Input: part model. Units: mm. Frame: model coordinates. Face numbers are marked on the shaded views. A direction names the side the tool comes from. Round coordinates to 2 decimals unless told otherwise and drop trailing zeros. Order: outer loops, then holes, each group sorted by start corner. A loop starts at its lowest first (then second) coordinate and runs counter-clockwise, first axis right, second up. Notation, with made-up numbers: (38, 22) -> (84, 22) arc R32 ccw to (84, 60) -> close; hole circle Ø1 at (86.5, 6.5). An arc over 180 degrees is marked (long way). Use a Markdown table: item, result.
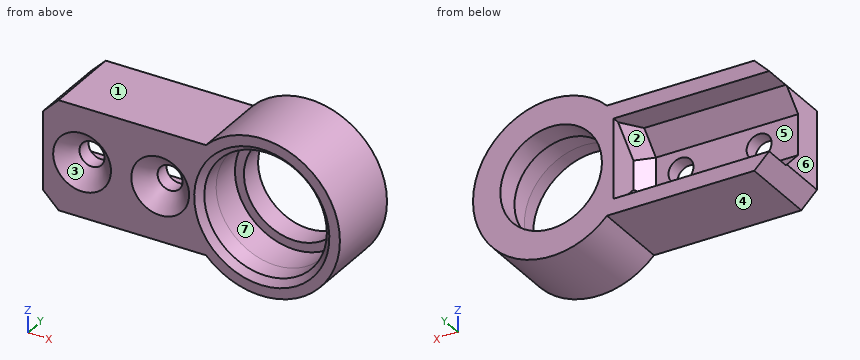
from build123d import *

# Parameters (mm, degrees)
BOSS_EXTRU_1_DEPTH      = 10
ESQUISSE2_W             = 10.2
ESQUISSE2_H             = 6
ENL_V_MAT_EXTRU_1_DEPTH = 20
CHANFREIN1_SIZE         = 2.5
CHANFREIN2_SIZE         = 1.8
ESQUISSE3_R             = 6.5
ENL_V_MAT_EXTRU_2_DEPTH = 32.368774283
ESQUISSE4_R             = 7.65
ENL_V_MAT_EXTRU_3_DEPTH = 7
CHANFREIN3_SIZE         = 1
ESQUISSE5_R             = 1.6
ENL_V_MAT_EXTRU_4_DEPTH = 7
CHANFREIN4_SIZE         = 2.1
CHANFREIN5_SIZE         = 2
CHANFREIN6_SIZE         = 2
CHANFREIN6_SIZE2        = 0.271180531


with BuildPart() as part:
    # Esquisse1 → Boss.-Extru.1 (new body)
    with BuildSketch(Plane(origin=(0, 0, 0), x_dir=(1, 0, 0), z_dir=(0, 1, 0))):
        with BuildLine():
            Line((-28, -7), (-7.141428429, -7))
            ThreePointArc((-7.141428429, -7), (10, 0), (-7.141428429, 7))
            Line((-7.141428429, 7), (-28, 7))
            Line((-28, 7), (-28, -7))
        make_face()
    extrude(amount=BOSS_EXTRU_1_DEPTH)

    # Esquisse2 → Enlèv. mat.-Extru.1 (cut)
    with BuildSketch(Plane.ZY.offset(28)):
        with Locations((0, 7)):
            Rectangle(ESQUISSE2_W, ESQUISSE2_H)
    extrude(amount=-ENL_V_MAT_EXTRU_1_DEPTH, mode=Mode.SUBTRACT)

    # Chanfrein1
    chanfrein1_edges = [part.edges().sort_by_distance(p)[0] for p in [
        (-18, 4, -5.1),
        (-18, 4, 5.1),
    ]]
    chamfer(chanfrein1_edges, length=CHANFREIN1_SIZE)

    # Chanfrein2
    chanfrein2_edges = [part.edges().sort_by_distance(p)[0] for p in [
        (-8, 4, 0),
        (-8, 5.25, -3.85),
        (-8, 5.25, 3.85),
    ]]
    chamfer(chanfrein2_edges, length=CHANFREIN2_SIZE)

    # Esquisse3 → Enlèv. mat.-Extru.2 (cut, through all)
    with BuildSketch(Plane.XZ):
        with Locations(Location((0, 0, 0), (0, 0, 270))):
            Circle(ESQUISSE3_R)
    extrude(amount=-ENL_V_MAT_EXTRU_2_DEPTH, mode=Mode.SUBTRACT)

    # Esquisse4 → Enlèv. mat.-Extru.3 (cut)
    with BuildSketch(Plane.XZ):
        with Locations(Location((0, 0, 0), (0, 0, 270))):
            Circle(ESQUISSE4_R)
    extrude(amount=-ENL_V_MAT_EXTRU_3_DEPTH, mode=Mode.SUBTRACT)

    # Chanfrein3
    chanfrein3_edges = [part.edges().sort_by_distance(p)[0] for p in [
        (0, 0, 7.65),
    ]]
    chamfer(chanfrein3_edges, length=CHANFREIN3_SIZE)

    # Esquisse5 → Enlèv. mat.-Extru.4 (cut)
    with BuildSketch(Plane.XZ):
        with Locations(Location((-23, 0, 0), (0, 0, 270))):
            Circle(ESQUISSE5_R)
        with Locations(Location((-13, 0, 0), (0, 0, 270))):
            Circle(ESQUISSE5_R)
    extrude(amount=-ENL_V_MAT_EXTRU_4_DEPTH, mode=Mode.SUBTRACT)

    # Chanfrein4
    chanfrein4_edges = [part.edges().sort_by_distance(p)[0] for p in [
        (-23, 0, 1.6),
        (-13, 0, 1.6),
    ]]
    chamfer(chanfrein4_edges, length=CHANFREIN4_SIZE)

    # Chanfrein5
    chanfrein5_edges = [part.edges().sort_by_distance(p)[0] for p in [
        (-28, 5, -7),
        (-28, 5, 7),
    ]]
    chamfer(chanfrein5_edges, length=CHANFREIN5_SIZE)

    # Chanfrein6
    chanfrein6_edges = [part.edges().sort_by_distance(p)[0] for p in [
        (0, 1, 7.65),
    ]]
    chanfrein6_side = [part.faces().sort_by_distance(p)[0] for p in [
        (0, 4, 7.65),
    ]]
    chamfer(chanfrein6_edges, length=CHANFREIN6_SIZE, length2=CHANFREIN6_SIZE2, reference=chanfrein6_side[0])


solid = part.part
1) Cut plane A-A on x = -23. Return loops of the section in (y, z).
Results found:
| item | result |
|---|---|
| outline | (0, -7) -> (10, -7) -> (10, -5.1) -> (6.5, -5.1) -> (4, -2.6) -> (4, -1.6) -> (2.1, -1.6) -> (0, -3.7) -> close; (0, 3.7) -> (2.1, 1.6) -> (4, 1.6) -> (4, 2.6) -> (6.5, 5.1) -> (10, 5.1) -> (10, 7) -> (0, 7) -> close |
2) Line query: L1, parallel to X at y = 3.1, z = 0; L2, parallel to X at y = 7.75, z = 0; L3, parallel to Z at x = -18.5, y = 7. Output: solid intervals per line, ascending. Write a range as [from, to].
Results found:
| item | result |
|---|---|
| L1 | x = [-28, -24.6], [-21.4, -14.6], [-11.4, -7.65], [7.65, 10] |
| L2 | x = [-8, -6.5], [6.5, 10] |
| L3 | z = [-7, -5.1], [5.1, 7] |
3) Cut plane B-B on z = 0. Count the separate pieces of the cut face and the enclosed holes in it, and give its area (3 significant figures).
Results found:
| item | result |
|---|---|
| separate pieces | 4 |
| enclosed holes | 0 |
| area | 79.7 mm² |
4) Set-up query: the marked faces 4, 5, 6 and 7. Return all of +Z, -Z, +X, -X, +Y, -Y with unobstructed straight access to the full face (end or side cutting, diameter ignored); none if empty.
Results found:
| item | result |
|---|---|
| face 4 | -Z, -X, +Y, -Y |
| face 5 | -X, +Y |
| face 6 | +Z, -Z, -X, +Y, -Y |
| face 7 | -Y |
5) Pull-direction query (X, two-part tool) for the marked faces 1, 2 and 3; classes: +X half, -X half, draft (parallel to the pull), parting line (faces both ways), or undercut.
Results found:
| item | result |
|---|---|
| face 1 | draft |
| face 2 | -X half |
| face 3 | undercut |
6) Pin query (flat end, axial travel): pin 1 Ø4 at (x, z) = (-23, 0) entering from +Y; pin 2 Ø1 at (x, y) = (-16, 8.5) entering from -Z; pin 3 Ø6 at (x, y) = (-6, 8.5) entering from +Z. Return the tip coordinate at first contact, or that it passes through.
Results found:
| item | result |
|---|---|
| pin 1 | stops at y = 4 |
| pin 2 | stops at z = -7 |
| pin 3 | stops at z = 9.54 |
